```python
from build123d import *

# Parameters (mm, degrees)
F0_W     = 58
F0_H     = 39
F1_DEPTH = 14
F2_W     = 58
F2_H     = 39
F2_W_2   = 7
F2_H_2   = 10
F3_DEPTH = 13
F4_R     = 1
F5_DEPTH = 25


with BuildPart() as f1:
    # F0 (on Top) → F1 (new body)
    with BuildSketch(Plane.XY):
        Rectangle(F0_W, F0_H)
    extrude(amount=F1_DEPTH)

    # F2 (on face) → F3 (cut)
    with BuildSketch(Plane.XY.offset(14)):
        Rectangle(F2_W, F2_H)
        with Locations((-21.244489, -3.62447)):
            Rectangle(F2_W_2, F2_H_2, mode=Mode.SUBTRACT)
        with Locations((-11.244526, -3.597112)):
            Rectangle(F2_W_2, F2_H_2, mode=Mode.SUBTRACT)
        with Locations((-1.244564, -3.569755)):
            Rectangle(F2_W_2, F2_H_2, mode=Mode.SUBTRACT)
        with Locations((8.755399, -3.542397)):
            Rectangle(F2_W_2, F2_H_2, mode=Mode.SUBTRACT)
        with Locations((18.755362, -3.515039)):
            Rectangle(F2_W_2, F2_H_2, mode=Mode.SUBTRACT)
    extrude(amount=-F3_DEPTH, mode=Mode.SUBTRACT)

    # F4 (on face) → F5 (cut)
    with BuildSketch(Plane.XY.offset(1)):
        with Locations((-27, 17.5)):
            Circle(F4_R)
        with Locations((-27, -17.5)):
            Circle(F4_R)
        with Locations((27, -17.5)):
            Circle(F4_R)
        with Locations((27, 17.5)):
            Circle(F4_R)
    extrude(amount=-F5_DEPTH, mode=Mode.SUBTRACT)


solid = f1.part
```
Geometry check sheet. Reference: the model listing, model coordinates, mm. A direction names the side the tool comes from. Round coordinates to 2 decimals unless told otherwise and drop trailing zeros. Loops run counter-clockwise (first coordinate to the right, second up) from the corner with the lowest first, then second, coordinate; pieces in that order, holes last. Notation, with made-up numbers: (0, -16) - (15, -16) arc R14 ccw to (15, 11) - close; hole circle Ø6 at (55.5, -1). An arc over 180 degrees is marked (long way). Use a Markdown table: item, result.
Q1. Go/stop test with flat-tipped pins: P1, Ø8, axis at y = -3.5, z = 4.5, coming from the +X side; P2, Ø4, axis at x = -8.5, z = 8.5, coming from the +Y side; P3, Ø2, axis at x = 18, z = 7, coming from the -Y side; P4, Ø8, axis at y = -0.5, z = 7.5, coming from the -X side. Record where each tip stops, or that it passes through.
Solutions:
| item | result |
|---|---|
| P1 | stops at x = 29 |
| P2 | stops at y = 1.4 |
| P3 | stops at y = -8.52 |
| P4 | stops at x = -24.74 |
Q2. Draft check along X on faces 1 (the flat face through (-17.744, -4, 8)), 2 (the flat face through (9, -8.542, 8)), 3 (the flat face through (5.255, -4, 8)), 4 (the flat face through (22.255, -4, 8)). Enter one of: released by +X, released by -X, zero draft, split by the parting line, or undercut.
Solutions:
| item | result |
|---|---|
| face 1 | undercut |
| face 2 | zero draft |
| face 3 | undercut |
| face 4 | released by +X |
Q3. Cross-section at C-C on x = -27. Record the cut outline in (y, z).
Solutions:
| item | result |
|---|---|
| outline | (-19.5, 0) - (-18.5, 0) - (-18.5, 1) - (-19.5, 1) - close; (-16.5, 0) - (16.5, 0) - (16.5, 1) - (-16.5, 1) - close; (18.5, 0) - (19.5, 0) - (19.5, 1) - (18.5, 1) - close |
Q4. Cross-section at D-D on y = -5.5. Record the cut outline in (x, z), plus the area to 3 significant figures.
Solutions:
| item | result |
|---|---|
| outline | (-29, 0) - (29, 0) - (29, 1) - (22.26, 1) - (22.26, 14) - (15.26, 14) - (15.26, 1) - (12.26, 1) - (12.26, 14) - (5.26, 14) - (5.26, 1) - (2.26, 1) - (2.26, 14) - (-4.74, 14) - (-4.74, 1) - (-7.74, 1) - (-7.74, 14) - (-14.74, 14) - (-14.74, 1) - (-17.74, 1) - (-17.74, 14) - (-24.74, 14) - (-24.74, 1) - (-29, 1) - close |
| area | 513 mm2 |
Q5. Access from +Z, -Z, +X, -X, +Y, -Y to the whole of each face (thin tool, end or side, straight path). Record for faces 5 (the flat face through (-4.745, -4, 8)), 6 (the flat face through (-11, 1.403, 8)), 7 (the flat face through (19, 1.485, 8)).
Solutions:
| item | result |
|---|---|
| face 5 | +Z, +Y, -Y |
| face 6 | +Z, -X, +Y |
| face 7 | +Z, +X, -X, +Y |
Q6. Material ranges on line 1 (Y direction, x = 27, z = 0.7); line 2 (X direction, y = -4, z = 7.75); line 3 (Z direction, x = 0, y = -13.5), recorded low to high.
Solutions:
| item | result |
|---|---|
| line 1 | y = -19.5 to -18.5, -16.5 to 16.5, 18.5 to 19.5 |
| line 2 | x = -24.74 to -17.74, -14.74 to -7.74, -4.74 to 2.26, 5.26 to 12.26, 15.26 to 22.26 |
| line 3 | z = 0 to 1 |
Q7. Cross-section at A-A on z = 9.25. Record the cut outline in (x, y).
Solutions:
| item | result |
|---|---|
| outline | (-24.74, -8.62) - (-17.74, -8.62) - (-17.74, 1.38) - (-24.74, 1.38) - close; (-14.74, -8.6) - (-7.74, -8.6) - (-7.74, 1.4) - (-14.74, 1.4) - close; (-4.74, -8.57) - (2.26, -8.57) - (2.26, 1.43) - (-4.74, 1.43) - close; (5.26, -8.54) - (12.26, -8.54) - (12.26, 1.46) - (5.26, 1.46) - close; (15.26, -8.52) - (22.26, -8.52) - (22.26, 1.48) - (15.26, 1.48) - close |
Q8. Cross-section at B-B on y = -17.5. Record the cut outline in (x, z).
Solutions:
| item | result |
|---|---|
| outline | (-29, 0) - (-28, 0) - (-28, 1) - (-29, 1) - close; (-26, 0) - (26, 0) - (26, 1) - (-26, 1) - close; (28, 0) - (29, 0) - (29, 1) - (28, 1) - close |
